The listing builds one solid part. Answer for the finished solid, in the listing's coordinates (mm). Face numbers are marked on the shaded views. A direction names the side the tool comes from. Round coordinates to 2 decimals unless told otherwise and drop trailing zeros. Order: outer loops, then holes, each group sorted by start corner. A loop starts at its lowest first (then second) coordinate and runs counter-clockwise, first axis right, second up. Notation, with made-up numbers: M 71.5,-11.75 L 76.5,-11.75 A22 cw 76.5,12.25 Z; hole C -32.5,1.25 d3. An arc over 180 degrees is marked long. Write item = value, one per line. Start each with the question number.
(1) Straight lines are drawn through the part: probe 1 along X at (y, z) = (-23.75, 5); probe 2 along Z at (x, y) = (14.5, 8); probe 3 along X at (y, z) = (-5.5, -0.5). For each, find the intervals that lie inside material, in ascending order. Write a range as from..to.
(2) A cutting plane is placed at B-B, the plane z = 5. Determine the outline of the cut face in (x, y), and give its area (3 significant figures).
(3) A cutting plane is placed at C-C, the plane x = -6.5. Determine the outline of the cut face in (y, z), and give its area (3 significant figures).
(4) A cutting plane is placed at A-A, the plane y = 0. Determine the outline of the cut face in (x, z), and give its area (3 significant figures).
(5) Each of these flat-tipped pins is pushed along its axis until it touches: pin 1 (6 mm diameter, centred on x = -16.26, y = 16.26, fed in from +Z); pin 2 (4 mm diameter, centred on x = 14, z = 5, fed in from +Y). Where does it stop, or does it pass through?
(6) Which of the six approach directions +Z, -Z, +X, -X, +Y, -Y give full straight-line access (tool end or side, diameter ignored) to the marked faces 1 and 2?
(7) A cutting plane is placed at D-D, the plane y = -8.5. Determine the outline of the cut face in (x, z), and give its area (3 significant figures).
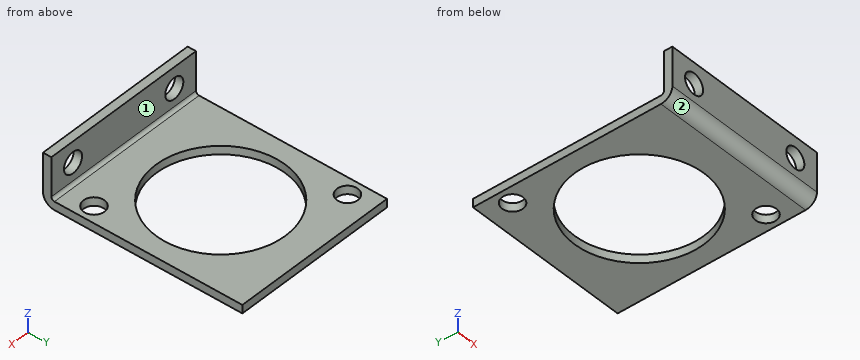
from build123d import *

# Parameters (mm, degrees)
SKETCH1_W          = 40
SKETCH1_H          = 45
BASE_FLANGE1_DEPTH = 2
SKETCH8_R          = 15.5
CUT_EXTRUDE5_DEPTH = 31.170349683
SKETCH9_R          = 2.5
CUT_EXTRUDE6_DEPTH = 31.170349683
EDGE_FLANGE1_DEPTH = 40
SKETCH13_R         = 2.5
CUT_EXTRUDE7_DEPTH = 53.714162988


# Sheet-metal steps are written as plain solids
with BuildPart() as part:
    # Sketch1 → Base-Flange1 (new body)
    with BuildSketch(Plane.XY):
        Rectangle(SKETCH1_W, SKETCH1_H)
    extrude(amount=-BASE_FLANGE1_DEPTH)

    # Sketch8 → Cut-Extrude5 (cut, through all)
    with BuildSketch(Plane.XY):
        Circle(SKETCH8_R)
    extrude(amount=-CUT_EXTRUDE5_DEPTH, mode=Mode.SUBTRACT)

    # Sketch9 → Cut-Extrude6 (cut, through all)
    with BuildSketch(Plane.XY):
        with Locations((-16.263455967, 16.263455967)):
            Circle(SKETCH9_R)
        with Locations((16.263455967, -16.263455967)):
            Circle(SKETCH9_R)
    extrude(amount=-CUT_EXTRUDE6_DEPTH, mode=Mode.SUBTRACT)

    # Edge-Flange1 section (across the edge) → Edge-Flange1 (add)
    with BuildSketch(Plane(origin=(-20, -23.2366, 0), x_dir=(0, 1, 0), z_dir=(1, 0, 0))):
        with BuildLine():
            Line((-2, 0.7366), (-2, 10))
            Line((-2, 10), (0, 10))
            Line((0, 10), (0, 0.7366))
            ThreePointArc((0, 0.7366), (0.215745145, 0.215745145), (0.7366, 0))
            Line((0.7366, 0), (0.7366, -2))
            ThreePointArc((0.7366, -2), (-1.198468417, -1.198468417), (-2, 0.7366))
        make_face()
    extrude(amount=EDGE_FLANGE1_DEPTH)

    # Sketch13 → Cut-Extrude7 (cut, through all)
    with BuildSketch(Plane.XZ.offset(25.2366)):
        with Locations(Location((-14, 5, 0), (0, 0, 270))):
            Circle(SKETCH13_R)
        with Locations(Location((14, 5, 0), (0, 0, 270))):
            Circle(SKETCH13_R)
    extrude(amount=-CUT_EXTRUDE7_DEPTH, mode=Mode.SUBTRACT)


solid = part.part
Reported:
q1.probe_1 = -20..-16.5, -11.5..11.5, 16.5..20
q1.probe_2 = -2..0
q1.probe_3 = -20..-14.49, 14.49..20
q2.outline = M -20,-25.24 L -16.5,-25.24 L -16.5,-23.24 L -20,-23.24 Z; M -11.5,-25.24 L 11.5,-25.24 L 11.5,-23.24 L -11.5,-23.24 Z; M 16.5,-25.24 L 20,-25.24 L 20,-23.24 L 16.5,-23.24 Z
q2.area = 60.0 mm²
q3.outline = M -25.24,0.74 A2.74 ccw -22.5,-2 L -14.07,-2 L -14.07,0 L -22.5,0 A0.74 cw -23.24,0.74 L -23.24,10 L -25.24,10 Z; M 14.07,-2 L 22.5,-2 L 22.5,0 L 14.07,0 Z
q3.area = 57.7 mm²
q4.outline = M -20,-2 L -15.5,-2 L -15.5,0 L -20,0 Z; M 15.5,-2 L 20,-2 L 20,0 L 15.5,0 Z
q4.area = 18.0 mm²
q5.pin_1 = 0
q5.pin_2 = through
q6.face_1 = +Z, +X, -X, +Y
q6.face_2 = -Z, +X, -X, -Y
q7.outline = M -20,-2 L -12.96,-2 L -12.96,0 L -20,0 Z; M 12.96,-2 L 20,-2 L 20,0 L 12.96,0 Z
q7.area = 28.2 mm²
